```python
from build123d import *

# Parameters (mm, degrees)
SKETCH1_W            = 355
SKETCH1_H            = 320
BOSS_EXTRUDE1_DEPTH  = 320
SKETCH9_W            = 296
SKETCH9_H            = 296
CUT_EXTRUDE3_DEPTH   = 345
SKETCH10_W           = 308
SKETCH10_H           = 308
CUT_EXTRUDE4_DEPTH   = 11
SKETCH11_W           = 280
SKETCH11_H           = 210
CUT_EXTRUDE5_DEPTH   = 20
SKETCH12_W           = 285
SKETCH12_H           = 35
BOSS_EXTRUDE4_DEPTH  = 17
SKETCH14_W           = 285
SKETCH14_H           = 35
BOSS_EXTRUDE5_DEPTH  = 17
SKETCH15_W           = 328
SKETCH15_H           = 35
BOSS_EXTRUDE6_DEPTH  = 17
SKETCH16_W           = 35
SKETCH16_H           = 300
BOSS_EXTRUDE7_DEPTH  = 5
SKETCH18_W           = 20
SKETCH18_H           = 300
BOSS_EXTRUDE10_DEPTH = 39


with BuildPart() as part:
    # Sketch1 → Boss-Extrude1 (new body)
    with BuildSketch(Plane(origin=(0, 0, 0), x_dir=(1, 0, 0), z_dir=(0, 1, 0))):
        with Locations((177.5, 160)):
            Rectangle(SKETCH1_W, SKETCH1_H)
    extrude(amount=BOSS_EXTRUDE1_DEPTH)

    # Sketch9 → Cut-Extrude3 (cut)
    with BuildSketch(Plane(origin=(355, 0, 0), x_dir=(0, 0, -1), z_dir=(1, 0, 0))):
        with Locations((160, 160)):
            Rectangle(SKETCH9_W, SKETCH9_H)
    extrude(amount=-CUT_EXTRUDE3_DEPTH, mode=Mode.SUBTRACT)

    # Sketch10 → Cut-Extrude4 (cut)
    with BuildSketch(Plane(origin=(355, 0, 0), x_dir=(0, 0, -1), z_dir=(1, 0, 0))):
        with Locations((160, 160)):
            Rectangle(SKETCH10_W, SKETCH10_H)
    extrude(amount=-CUT_EXTRUDE4_DEPTH, mode=Mode.SUBTRACT)

    # Sketch11 → Cut-Extrude5 (cut)
    with BuildSketch(Plane.XZ):
        with Locations((165, -160)):
            Rectangle(SKETCH11_W, SKETCH11_H)
    extrude(amount=-CUT_EXTRUDE5_DEPTH, mode=Mode.SUBTRACT)

    # Sketch12 → Boss-Extrude4 (add)
    with BuildSketch(Plane.XZ):
        with Locations((162.5, -27.5)):
            Rectangle(SKETCH12_W, SKETCH12_H)
    extrude(amount=BOSS_EXTRUDE4_DEPTH)

    # Sketch14 → Boss-Extrude5 (add)
    with BuildSketch(Plane.XZ):
        with Locations((162.5, -292.5)):
            Rectangle(SKETCH14_W, SKETCH14_H)
    extrude(amount=BOSS_EXTRUDE5_DEPTH)

    # Sketch15 → Boss-Extrude6 (add)
    with BuildSketch(Plane.XZ.offset(17)):
        with Locations((184, -27.5)):
            Rectangle(SKETCH15_W, SKETCH15_H)
        with Locations((184, -292.5)):
            Rectangle(SKETCH15_W, SKETCH15_H)
    extrude(amount=BOSS_EXTRUDE6_DEPTH)

    # Sketch16 → Boss-Extrude7 (add)
    with BuildSketch(Plane.XZ.offset(34)):
        with Locations((37.5, -160)):
            Rectangle(SKETCH16_W, SKETCH16_H)
    extrude(amount=BOSS_EXTRUDE7_DEPTH)

    # Sketch18 → Boss-Extrude10 (add)
    with BuildSketch(Plane.XZ):
        with Locations((10, -160)):
            Rectangle(SKETCH18_W, SKETCH18_H)
    extrude(amount=BOSS_EXTRUDE10_DEPTH)


solid = part.part
```
Source: CAD feature listing. Evaluate the final solid. Frame: model axes, mm. A direction names the side the tool comes from. Round coordinates to 2 decimals unless told otherwise and drop trailing zeros. Loops run counter-clockwise (first coordinate to the right, second up) from the corner with the lowest first, then second, coordinate; pieces in that order, holes last.
1. Access query for faces 1 (the flat face through (305, 6, -161)), 2 (the flat face through (350, 158, -6)), 3 (the flat face through (199, -34, -27)), 4 (the flat face through (25, 6, -161)). Directions: +Z, -Z, +X, -X, +Y, -Y. A direction counts if a zero-diameter tool reaches every point of the face in a straight line with its end or side. Return the directions, or none.
2. Contact query for flat-ended pins moving along their axis: pin 1 (13.5 mm diameter, centred on y = -23.5, z = -30.5, fed in from +X); pin 2 (12 mm diameter, centred on y = 130.5, z = -181.5, fed in from +X); pin 3 (4 mm diameter, centred on y = -36.5, z = -178.5, fed in from +X). Output: stop coordinate, or through.
3. Section query B-B on x = 46.5. Output: boundary loops of the cut face in (y, z).
4. Ray query, L1, parallel to Z at x = 85.5, y = 238; L2, parallel to Y at x = 103, z = -45.5; L3, parallel to Y at x = 53.5, z = -246. Return the intervals inside material, ascending.
5. Section query C-C on y = 111.5. Output: boundary loops of the cut face in (x, z).
6. Mould query, pull axis Z, two halves, no side actions, for faces 5 (the flat face through (350, 314, -158)), 6 (the flat face through (175, 320, -162)), 7 (the flat face through (172, -19, -310)). Classes: released by +Z, released by -Z, zero draft, split by the parting line, or undercut.
7. Section query D-D on x = 249.5. Output: boundary loops of the cut face in (y, z).
8. Section query A-A on z = -251.5. Output: boundary loops of the cut face in (x, y).
Answers below:
1. face 1: -Y
1. face 2: +X
1. face 3: +Z, -Z, +X, -Y
1. face 4: none
2. pin 1: stops at x = 348
2. pin 2: stops at x = 10
2. pin 3: stops at x = 55
3. outline: (-39, -310) - (0, -310) - (0, -320) - (320, -320) - (320, 0) - (0, 0) - (0, -10) - (-39, -10) - close; hole (-34, -275) - (0, -275) - (0, -265) - (12, -265) - (12, -308) - (308, -308) - (308, -12) - (12, -12) - (12, -55) - (0, -55) - (0, -45) - (-34, -45) - close
4. L1: z = -320 to -308, -12 to 0
4. L2: y = 0 to 12, 308 to 320
4. L3: y = -39 to -34, 308 to 320
5. outline: (0, -320) - (355, -320) - (355, -314) - (344, -314) - (344, -308) - (10, -308) - (10, -12) - (344, -12) - (344, -6) - (355, -6) - (355, 0) - (0, 0) - close
6. face 5: undercut
6. face 6: zero draft
6. face 7: released by -Z
7. outline: (-34, -310) - (0, -310) - (0, -320) - (320, -320) - (320, 0) - (0, 0) - (0, -10) - (-34, -10) - (-34, -45) - (0, -45) - (0, -55) - (12, -55) - (12, -12) - (308, -12) - (308, -308) - (12, -308) - (12, -265) - (0, -265) - (0, -275) - (-34, -275) - close
8. outline: (0, -39) - (55, -39) - (55, -34) - (20, -34) - (20, 0) - (25, 0) - (25, 12) - (10, 12) - (10, 308) - (344, 308) - (344, 314) - (355, 314) - (355, 320) - (0, 320) - close; (305, 0) - (355, 0) - (355, 6) - (344, 6) - (344, 12) - (305, 12) - close
